```python
from build123d import *

# Parameters (mm, degrees)
EXTRUDE_1_DEPTH = 3
SKETCH_2_R      = 11
SKETCH_2_R_2    = 1.65
EXTRUDE_2_DEPTH = 3
EXTRUDE_3_DEPTH = 3


with BuildPart() as part:
    # 草图1 → 凸台-拉伸1 (new body)
    with BuildSketch(Plane(origin=(0, 0, 0), x_dir=(1, 0, 0), z_dir=(0, 1, 0))):
        Polygon((19.5, -53), (25, -47.5), (25, 0), (-25, 0), (-25, -47.5), (-19.5, -53), align=None)
        with BuildLine():
            Line((17.15, -12.15), (17.15, -41.85))
            ThreePointArc((17.15, -41.85), (15, -44), (12.85, -41.85))
            Line((12.85, -41.85), (12.85, -12.15))
            ThreePointArc((12.85, -12.15), (15, -10), (17.15, -12.15))
        make_face(mode=Mode.SUBTRACT)
        with BuildLine():
            Line((-17.15, -12.15), (-17.15, -41.85))
            ThreePointArc((-17.15, -41.85), (-15, -44), (-12.85, -41.85))
            Line((-12.85, -41.85), (-12.85, -12.15))
            ThreePointArc((-12.85, -12.15), (-15, -10), (-17.15, -12.15))
        make_face(mode=Mode.SUBTRACT)
    extrude(amount=-EXTRUDE_1_DEPTH)

    # 草图2 → 凸台-拉伸2 (add)
    with BuildSketch(Plane(origin=(0, 0, 0), x_dir=(-1, 0, 0), z_dir=(0, 0, -1))):
        Polygon((-25.5, -3), (25.5, -3), (25.5, 42.5), (20, 48), (-20, 48), (-25.5, 42.5), align=None)
        with Locations((0, 27)):
            Circle(SKETCH_2_R, mode=Mode.SUBTRACT)
        with Locations((-15.5, 42.5)):
            Circle(SKETCH_2_R_2, mode=Mode.SUBTRACT)
        with Locations((-15.5, 11.5)):
            Circle(SKETCH_2_R_2, mode=Mode.SUBTRACT)
        with Locations((15.5, 11.5)):
            Circle(SKETCH_2_R_2, mode=Mode.SUBTRACT)
        with Locations((15.5, 42.5)):
            Circle(SKETCH_2_R_2, mode=Mode.SUBTRACT)
    extrude(amount=EXTRUDE_2_DEPTH)

    # 草图4 → 凸台-拉伸3 (add)
    with BuildSketch(Plane(origin=(25.5, 0, 0), x_dir=(0, 0, -1), z_dir=(1, 0, 0))):
        with BuildLine():
            Line((-1.707106781, 13.292893219), (-13.292893219, 1.707106781))
            ThreePointArc((-13.292893219, 1.707106781), (-13.50966597, 0.617316568), (-12.585786438, 0))
            Line((-12.585786438, 0), (-1, 0))
            ThreePointArc((-1, 0), (-0.292893219, 0.292893219), (0, 1))
            Line((0, 1), (0, 12.585786438))
            ThreePointArc((0, 12.585786438), (-0.617316568, 13.50966597), (-1.707106781, 13.292893219))
        make_face()
    extrude_3 = extrude(amount=-EXTRUDE_3_DEPTH)

    # 镜向1: 凸台-拉伸3 across plane
    add(extrude_3.mirror(Plane(origin=(0, 0, 0), x_dir=(0, 0, 1), z_dir=(1, 0, 0))))


solid = part.part
```
Here's how the part is built. I have some questions about the finished solid (model axes, mm). A direction names the side the tool comes from. Round coordinates to 2 decimals unless told otherwise and drop trailing zeros. Order: outer loops, then holes, each group sorted by start corner. A loop starts at its lowest first (then second) coordinate and runs counter-clockwise, first axis right, second up. Notation, with made-up numbers: M 83,-25.75 L 99,-25.75 A13 cw 99,-8.75 Z; hole C 58,88 d11. An arc over 180 degrees is marked long. Answer in a Markdown table with one row per item.
Item 1: Imagine slicing it at C-C, the plane z = 34.5. Write out the boundary of the cut face in (x, y).
A:
| item | result |
|---|---|
| outline | M -25,-3 L -17.15,-3 L -17.15,0 L -25,0 Z; M -12.85,-3 L 12.85,-3 L 12.85,0 L -12.85,0 Z; M 17.15,-3 L 25,-3 L 25,0 L 17.15,0 Z |
Item 2: For faces 1 (the face through (0, -1, 53)), 2 (the face through (-15, -1, 10)), 3 (the face through (23, 45, -1)), 4 (the face through (25, -1, 24)), 5 (the face through (-25, -1, 23)), which set-ups out of +Z, -Z, +X, -X, +Y, -Y let a thin tool reach every point of the face, with its end or its side?
A:
| item | result |
|---|---|
| face 1 | +Z, +X, -X, +Y, -Y |
| face 2 | +Y, -Y |
| face 3 | +Z, -Z, +X, +Y |
| face 4 | +Z, +X, -Y |
| face 5 | +Z, -X, -Y |
Item 3: Imagine slicing it at A-A, the plane y = 11.5. Write out the boundary of the cut face in (x, z), and give its area (3 significant figures).
A:
| item | result |
|---|---|
| outline | M -25.5,-3 L -17.15,-3 L -17.15,0 L -22.5,0 L -22.5,3.5 L -25.5,3.5 Z; M -13.85,-3 L 13.85,-3 L 13.85,0 L -13.85,0 Z; M 17.15,-3 L 25.5,-3 L 25.5,3.5 L 22.5,3.5 L 22.5,0 L 17.15,0 Z |
| area | 154 mm2 |
Item 4: Thinking about a two-plate mould opening in Y: for faces 6 (the face through (-12.85, -1, 27)), 7 (the face through (24.021, 0.633, 13.516)), 8 (the face through (0, -3, 25)), 9 (the face through (14.61, 43.89, -1.48)), which applies, +Y half, -Y half, draft (parallel to the pull), parting line (faces both ways), or undercut?
A:
| item | result |
|---|---|
| face 6 | draft |
| face 7 | undercut |
| face 8 | -Y half |
| face 9 | undercut |
Item 5: Imagine slicing it at D-D, the plane x = 3. Write out the boundary of the cut face in (y, z).
A:
| item | result |
|---|---|
| outline | M -3,-3 L 16.42,-3 L 16.42,0 L 0,0 L 0,53 L -3,53 Z; M 37.58,-3 L 48,-3 L 48,0 L 37.58,0 Z |
Item 6: I'm going to push flat-ended pins straight in: pin 1 (0.9 mm diameter, centred on y = -1, z = 14.5, fed in from +X); pin 2 (15 mm diameter, centred on x = 10, z = 29, fed in from +Y); pin 3 (0.9 mm diameter, centred on y = -1, z = 24, fed in from -X); pin 4 (5.5 mm diameter, centred on x = -15.5, y = 42.5, fed in from -Z). Where does each tip first touch, or does it pass through?
A:
| item | result |
|---|---|
| pin 1 | stops at x = 25 |
| pin 2 | stops at y = 0 |
| pin 3 | stops at x = -25 |
| pin 4 | stops at z = -3 |
Item 7: Imagine slicing it at B-B, the plane y = 27. Write out the boundary of the cut face in (x, z).
A:
| item | result |
|---|---|
| outline | M -25.5,-3 L -11,-3 L -11,0 L -25.5,0 Z; M 11,-3 L 25.5,-3 L 25.5,0 L 11,0 Z |
Item 8: If I drill on L1, parallel to Y at x = -15.5, z = -2.3; L2, parallel to Y at x = 0, z = -1.75; L3, parallel to Z at x = -18, y = 14, over which ranges is the centre line in solid material (lowest first)? Write a range as from..to.
A:
| item | result |
|---|---|
| L1 | y = -3..9.85, 13.15..40.85, 44.15..48 |
| L2 | y = -3..16, 38..48 |
| L3 | z = -3..0 |
